The model under review builds one solid part; all positions refer to its coordinate system, in mm. Face numbers are marked on the shaded views. A direction names the side the tool comes from. Give positions to 0.01 mm unless a question says otherwise; leave off trailing zeros. Order: outer loops, then holes, each group sorted by start corner. A loop starts at its lowest first (then second) coordinate and runs counter-clockwise, first axis right, second up.
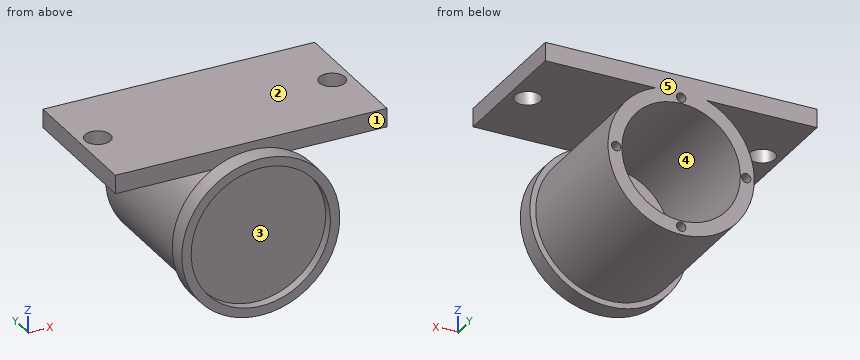
```python
from build123d import *

# Parameters (mm, degrees)
SKETCH1_R                 = 17
BOSS_EXTRUDE2_DEPTH       = 4
SHELL1_T                  = -2
SKETCH14_R                = 15.75
BOSS_EXTRUDE7_DEPTH       = 30
SHELL4_T                  = -3
BOSS_EXTRUDE12_DEPTH      = 3
BOSS_EXTRUDE12_DEPTH_BACK = 1
SKETCH16_W                = 58.499045292
SKETCH16_H                = 30
SKETCH17_R                = 2.75
CUT_EXTRUDE4_DEPTH        = 5
SKETCH18_R                = 1
CUT_EXTRUDE5_DEPTH        = 7


with BuildPart() as part:
    # Sketch1 → Boss-Extrude2 (new body)
    with BuildSketch(Plane(origin=(0, 0, 0), x_dir=(1, 0, 0), z_dir=(0, 1, 0))):
        with Locations(Location((0, 0, 0), (0, 0, 270))):
            Circle(SKETCH1_R)
    extrude(amount=BOSS_EXTRUDE2_DEPTH)

    # Shell1
    shell1_openings = [part.faces().sort_by_distance(p)[0] for p in [
        (0, 0, 0),
    ]]
    offset(amount=SHELL1_T, openings=shell1_openings, kind=Kind.INTERSECTION)

    # Sketch14 → Boss-Extrude7 (add)
    with BuildSketch(Plane(origin=(0, 4, 0), x_dir=(1, 0, 0), z_dir=(0, 1, 0))):
        with Locations(Location((0, 0, 0), (0, 0, 270))):
            Circle(SKETCH14_R)
    extrude(amount=BOSS_EXTRUDE7_DEPTH)

    # Shell4
    shell4_openings = [part.faces().sort_by_distance(p)[0] for p in [
        (0, 34, 0),
    ]]
    offset(amount=SHELL4_T, openings=shell4_openings, kind=Kind.INTERSECTION)

    # Sketch16 → Boss-Extrude12 (add, two sides: drawn at the far end of the back side and taken through both)
    with BuildSketch(Plane.XY.offset(15.75).offset(-BOSS_EXTRUDE12_DEPTH_BACK)):
        with Locations((0, 19)):
            Rectangle(SKETCH16_W, SKETCH16_H)
    extrude(amount=BOSS_EXTRUDE12_DEPTH + BOSS_EXTRUDE12_DEPTH_BACK)

    # Sketch17 → Cut-Extrude4 (cut)
    with BuildSketch(Plane.XY.offset(18.75)):
        with Locations((-25.244673943, 19)):
            Circle(SKETCH17_R)
        with Locations((25.244673943, 19)):
            Circle(SKETCH17_R)
    extrude(amount=-CUT_EXTRUDE4_DEPTH, mode=Mode.SUBTRACT)

    # Sketch18 → Cut-Extrude5 (cut)
    with BuildSketch(Plane(origin=(0, 34, 0), x_dir=(1, 0, 0), z_dir=(0, 1, 0))):
        with Locations(Location((0, 14, 0), (0, 0, 270))):
            Circle(SKETCH18_R)
        with Locations(Location((14, 0, 0), (0, 0, 270))):
            Circle(SKETCH18_R)
        with Locations(Location((0, -14, 0), (0, 0, 270))):
            Circle(SKETCH18_R)
        with Locations(Location((-14, 0, 0), (0, 0, 270))):
            Circle(SKETCH18_R)
    extrude(amount=-CUT_EXTRUDE5_DEPTH, mode=Mode.SUBTRACT)


solid = part.part
```
Item 1: Clearance check with flat-ended pins moving along their axes: pin 1 Ø12 at (x, y) = (-19, 13) entering from -Z; pin 2 Ø5 at (x, z) = (0.5, 3) entering from +Y; pin 3 Ø1.2 at (x, z) = (-14, 0) entering from +Y. State where each tip first meets the part, or that it passes through.
Values found:
pin 1: stops at z = -8.89
pin 2: stops at y = 5
pin 3: stops at y = 27
Item 2: Take a section at A-A (y = 19). Give the boundary of the cut face in (x, z), and give its area (3 significant figures).
Values found:
outline: (-29.25, 14.75) - (-27.99, 14.75) - (-27.99, 18.75) - (-29.25, 18.75) - close; (-22.49, 14.75) - (-5.52, 14.75) arc R15.75 ccw (long way) to (5.52, 14.75) - (22.49, 14.75) - (22.49, 18.75) - (-22.49, 18.75) - close; (27.99, 14.75) - (29.25, 14.75) - (29.25, 18.75) - (27.99, 18.75) - close; hole circle Ø25.5 at (0, 0)
area: 451 mm2
Item 3: For the marked faces 4 and 5, list the 3-axis set-ups (+Z, -Z, +X, -X, +Y, -Y) from which the entire face can be reached by the end or side of a thin tool; tool diameter is ignored.
Values found:
face 4: +Y
face 5: +Z, -Z, +X, -X, +Y
Item 4: Take a section at C-C (x = -11). Give the boundary of the cut face in (y, z).
Values found:
outline: (0, -12.96) - (4, -12.96) - (4, -11.27) - (34, -11.27) - (34, -6.45) - (5, -6.45) - (5, 6.45) - (34, 6.45) - (34, 11.27) - (4, 11.27) - (4, 12.96) - (0, 12.96) - (0, 10.2) - (2, 10.2) - (2, -10.2) - (0, -10.2) - close; (4, 14.75) - (34, 14.75) - (34, 18.75) - (4, 18.75) - close
Item 5: Draft analysis for pull direction Z (two halves, no side actions). For the marked faces 1, 2 and 3, state which applies: released by +Z, released by -Z, zero draft, split by the parting line, or undercut.
Values found:
face 1: zero draft
face 2: released by +Z
face 3: undercut
Item 6: Take a section at D-D (z = -14). Give the boundary of the cut face in (x, y).
Values found:
outline: (-9.64, 0) - (-5.39, 0) - (-5.39, 2) - (5.39, 2) - (5.39, 0) - (9.64, 0) - (9.64, 4) - (7.22, 4) - (7.22, 34) - (1, 34) - (1, 27) - (-1, 27) - (-1, 34) - (-7.22, 34) - (-7.22, 4) - (-9.64, 4) - close
Item 7: For line 1 (X direction, y = 31, z = 0); line 2 (Z direction, x = 0, y = 0.8); line 3 (Z direction, x = -0.5, y = 13), list the stretches that pass through material, from the lowest coordinate up.
Values found:
line 1: x = -15.75 to -15, -13 to -12.75, 12.75 to 13, 15 to 15.75
line 2: z = -17 to -15, 15 to 17
line 3: z = -15.74 to -12.74, 12.74 to 18.75
Item 8: Take a section at B-B (y = 7). Give the boundary of the cut face in (x, z).
Values found:
outline: (-29.25, 14.75) - (-5.52, 14.75) arc R15.75 ccw (long way) to (5.52, 14.75) - (29.25, 14.75) - (29.25, 18.75) - (-29.25, 18.75) - close; hole circle Ø25.5 at (0, 0)
